```python
from build123d import *

# Parameters (mm, degrees)
F0_R     = 50.8
F0_W     = 5.51793
F0_H     = 18.327414
F0_R_2   = 12.7
F0_W_2   = 18.327416
F0_H_2   = 8.868104
F0_W_3   = 5.320862
F0_H_3   = 18.130345
F0_W_4   = 13.991896
F0_H_4   = 14.780173
F1_DEPTH = 12.7


with BuildPart() as f1:
    # F0 (on Top) → F1 (new body)
    with BuildSketch(Plane.XY):
        Circle(F0_R)
        with Locations((-31.925172, -3.054569)):
            Rectangle(F0_W, F0_H, mode=Mode.SUBTRACT)
        Circle(F0_R_2, mode=Mode.SUBTRACT)
        with Locations((3.05457, -35.176811)):
            Rectangle(F0_W_2, F0_H_2, mode=Mode.SUBTRACT)
        with Locations((33.60026, -2.167758)):
            Rectangle(F0_W_3, F0_H_3, mode=Mode.SUBTRACT)
        with Locations((2.660431, 31.432501)):
            Rectangle(F0_W_4, F0_H_4, mode=Mode.SUBTRACT)
    extrude(amount=F1_DEPTH)


solid = f1.part
```
Read the model definition and answer for the solid it produces. Units are mm, in the model's axes. Round coordinates to 2 decimals unless told otherwise and drop trailing zeros. Write each loop counter-clockwise with the first axis right and the second up, starting at its lowest first coordinate (ties: lowest second). Pieces come first, ordered by that corner, then holes. Notation, with made-up numbers: (70, -16.5) - (129, -16.5) arc R5 ccw to (129, -8.5) - close; hole circle Ø6 at (35, -22). An arc over 180 degrees is marked (long way). One line per item, written item: value.
Q1. For a pull along X with two mould halves and no side action, classify faces 1 (the flat face through (11, -11, 12.7)), 2 (the flat face through (-32, -12.218, 6)), 3 (the cylindrical face through (-11.012, -49.592, 6.261)), 4 (the flat face through (36.261, -2, 6)) as pulls with the +X half, pulls with the -X half, needs draft (parallel to the pull), parting line crosses it, or undercut.
The answers:
face 1: needs draft
face 2: undercut
face 3: parting line crosses it
face 4: undercut
Q2. Find section D-D (y = -32.5). Determine the outline of the cut face in (x, z).
The answers:
outline: (-39.04, 0) - (-6.11, 0) - (-6.11, 12.7) - (-39.04, 12.7) - close; (12.22, 0) - (39.04, 0) - (39.04, 12.7) - (12.22, 12.7) - close
Q3. Straight lines are drawn through the part: line 1 (Y direction, x = -0.5, z = 10.5); line 2 (Y direction, x = 36, z = 9.75); line 3 (Y direction, x = -6, z = 4.25). For each, find the intervals that lie inside material, in ascending order. Write a range as from..to.
The answers:
line 1: y = -50.8..-39.61, -30.74..-12.69, 12.69..24.04, 38.82..50.8
line 2: y = -35.84..-11.23, 6.9..35.84
line 3: y = -50.44..-39.61, -30.74..-11.19, 11.19..50.44
Q4. Find section A-A (y = 0). Determine the outline of the cut face in (x, z), and give its area (3 significant figures).
The answers:
outline: (-50.8, 0) - (-34.68, 0) - (-34.68, 12.7) - (-50.8, 12.7) - close; (-29.17, 0) - (-12.7, 0) - (-12.7, 12.7) - (-29.17, 12.7) - close; (12.7, 0) - (30.94, 0) - (30.94, 12.7) - (12.7, 12.7) - close; (36.26, 0) - (50.8, 0) - (50.8, 12.7) - (36.26, 12.7) - close
area: 830 mm2
Q5. Find section C-C (x = 0). Determine the outline of the cut face in (y, z).
The answers:
outline: (-50.8, 0) - (-39.61, 0) - (-39.61, 12.7) - (-50.8, 12.7) - close; (-30.74, 0) - (-12.7, 0) - (-12.7, 12.7) - (-30.74, 12.7) - close; (12.7, 0) - (24.04, 0) - (24.04, 12.7) - (12.7, 12.7) - close; (38.82, 0) - (50.8, 0) - (50.8, 12.7) - (38.82, 12.7) - close
Q6. Each of these flat-tipped pins is pushed along its axis until it touches: P1, Ø3, axis at y = -39.5, z = 7, coming from the -X side; P2, Ø6, axis at x = -30.5, z = 5.5, coming from the -Y side; P3, Ø1.7, axis at x = -32.5, z = 6, coming from the +Y side. Where does it stop, or does it pass through?
The answers:
P1: stops at x = -33.71
P2: stops at y = -42.71
P3: stops at y = 39.74
Q7. Find section B-B (z = 5.5). Determine the outline of the cut face in (x, y).
The answers:
outline: circle Ø101.6 at (0, 0); hole (-34.68, -12.22) - (-29.17, -12.22) - (-29.17, 6.11) - (-34.68, 6.11) - close; hole circle Ø25.4 at (0, 0); hole (-6.11, -39.61) - (12.22, -39.61) - (12.22, -30.74) - (-6.11, -30.74) - close; hole (-4.34, 24.04) - (9.66, 24.04) - (9.66, 38.82) - (-4.34, 38.82) - close; hole (30.94, -11.23) - (36.26, -11.23) - (36.26, 6.9) - (30.94, 6.9) - close
